```python
from build123d import *

# Parameters (mm, degrees)
SKETCH1_W           = 101.6
SKETCH1_H           = 101.6
BOSS_EXTRUDE2_DEPTH = 116.84
SKETCH2_W           = 76.2
SKETCH2_H           = 55.88
CUT_EXTRUDE1_DEPTH  = 99.06
SKETCH3_W           = 111.76
SKETCH3_H           = 17.78
CUT_EXTRUDE2_DEPTH  = 96.52
SKETCH4_W           = 96.52
SKETCH4_H           = 96.52
CUT_EXTRUDE3_DEPTH  = 35.56
SKETCH5_R           = 1.0795
BOSS_EXTRUDE3_DEPTH = 29.464
SKETCH8_W           = 3.048
SKETCH8_H           = 91.44
CUT_EXTRUDE4_DEPTH  = 2.54
SKETCH10_W          = 2.54
SKETCH10_H          = 5.08
SKETCH10_H_2        = 5.198880867
BOSS_EXTRUDE4_DEPTH = 96.52


with BuildPart() as part:
    # Sketch1 → Boss-Extrude2 (new body)
    with BuildSketch(Plane.XY):
        with Locations((50.8, -50.8)):
            Rectangle(SKETCH1_W, SKETCH1_H)
    extrude(amount=BOSS_EXTRUDE2_DEPTH)

    # Sketch2 → Cut-Extrude1 (cut)
    with BuildSketch(Plane(origin=(101.6, 0, 0), x_dir=(0, 0, -1), z_dir=(1, 0, 0))):
        with Locations((-40.64, -50.8)):
            Rectangle(SKETCH2_W, SKETCH2_H)
    extrude(amount=-CUT_EXTRUDE1_DEPTH, mode=Mode.SUBTRACT)

    # Sketch3 → Cut-Extrude2 (cut)
    with BuildSketch(Plane(origin=(99.06, 0, 0), x_dir=(0, 0, -1), z_dir=(1, 0, 0))):
        with Locations((-58.42, -90.17)):
            Rectangle(SKETCH3_W, SKETCH3_H)
        with Locations((-58.42, -11.43)):
            Rectangle(SKETCH3_W, SKETCH3_H)
    extrude(amount=-CUT_EXTRUDE2_DEPTH, mode=Mode.SUBTRACT)

    # Sketch4 → Cut-Extrude3 (cut)
    with BuildSketch(Plane.XY.offset(116.84)):
        with Locations((50.8, -50.8)):
            Rectangle(SKETCH4_W, SKETCH4_H)
    extrude(amount=-CUT_EXTRUDE3_DEPTH, mode=Mode.SUBTRACT)

    # Sketch5 → Boss-Extrude3 (add)
    with BuildSketch(Plane.XY.offset(81.28)):
        with Locations((85.09, -41.91)):
            Circle(SKETCH5_R)
        with Locations((85.09, -69.85)):
            Circle(SKETCH5_R)
        with Locations((34.29, -26.67)):
            Circle(SKETCH5_R)
        with Locations((33.02, -74.93)):
            Circle(SKETCH5_R)
    extrude(amount=BOSS_EXTRUDE3_DEPTH)

    # Sketch8 → Cut-Extrude4 (cut)
    with BuildSketch(Plane.ZY):
        with Locations((112.776, -50.8)):
            Rectangle(SKETCH8_W, SKETCH8_H)
    extrude(amount=-CUT_EXTRUDE4_DEPTH, mode=Mode.SUBTRACT)

    # Sketch10 → Boss-Extrude4 (add)
    with BuildSketch(Plane(origin=(2.54, 0, 0), x_dir=(0, 0, -1), z_dir=(1, 0, 0))):
        with Locations((-115.57, -96.52)):
            Rectangle(SKETCH10_W, SKETCH10_H)
        with Locations((-109.982, -96.52)):
            Rectangle(SKETCH10_W, SKETCH10_H)
        with Locations((-115.57, -5.139440434)):
            Rectangle(SKETCH10_W, SKETCH10_H_2)
        with Locations((-109.982, -5.08)):
            Rectangle(SKETCH10_W, SKETCH10_H)
    extrude(amount=BOSS_EXTRUDE4_DEPTH)


solid = part.part
```
Work out the finished part from the listing and answer in its coordinate system (mm). A direction names the side the tool comes from. Coordinates: 2 decimals unless noted, no trailing zeros. Loops run counter-clockwise (first coordinate to the right, second up) from the corner with the lowest first, then second, coordinate; pieces in that order, holes last. Notation, with made-up numbers: M 46,-27 L 78,-27 A10 cw 78,-18 Z; hole C 51.25,59 d9. An arc over 180 degrees is marked long. Use CSV: the item, a comma, the result in double quotes. Start each with the question number.
(1) Given pin 1 Ø12 at (x, y) = (74, -37) entering from +Z; pin 2 Ø5.5 at (x, y) = (51, -15.5) entering from +Z; pin 3 Ø6 at (y, z) = (-48.5, 31) entering from +X, each flat-ended and moving along its own axis, determine where each tip first touches the part or whether it passes through.
(2) Find section C-C, the plane x = 91. Give the vertices of the cut face in (y, z).
(3) For a pull along Y with two mould halves and no side action, classify faces 4 (the face through (53, -78.74, 41)), 5 (the face through (50, 0, 58)), 6 (the face through (47, -96, 116.84)) as +Y half, -Y half, draft (parallel to the pull), parting line (faces both ways), or undercut.
(4) Find section B-B, the plane y = -35.5. Give the vertices of the cut face in (x, z).
(5) Find section D-D, the plane z = 40.5. Give the vertices of the cut face in (x, y).
(6) For faces 1 (the face through (53, -51, 2.54)), 2 (the face through (50, -50, 81.28)), 3 (the face through (50, -2.54, 56)), determine the directions among +Z, -Z, +X, -X, +Y, -Y from which every point of the face is accessible in a straight line to the end or side of a thin tool.
(7) Consider line 1 (Y direction, x = 10, z = 42.5); line 2 (Z direction, x = 33, y = -5.5); line 3 (X direction, y = -54, z = 91.5). Determine where each line is inside the solid, lowest interval first.
(8) Find section A-A, the plane z = 87. Give the vertices of the cut face in (x, y).
Recorded:
1,pin 1,"stops at z = 81.28"
1,pin 2,"stops at z = 2.54"
1,pin 3,"stops at x = 2.54"
2,outline,"M -101.6,0 L 0,0 L 0,116.84 L -7.74,116.84 L -7.74,114.3 L -2.54,114.3 L -2.54,111.25 L -7.62,111.25 L -7.62,108.71 L -2.54,108.71 L -2.54,2.54 L -20.32,2.54 L -20.32,81.28 L -81.28,81.28 L -81.28,2.54 L -99.06,2.54 L -99.06,108.71 L -93.98,108.71 L -93.98,111.25 L -99.06,111.25 L -99.06,114.3 L -93.98,114.3 L -93.98,116.84 L -101.6,116.84 Z; hole M -78.74,2.54 L -22.86,2.54 L -22.86,78.74 L -78.74,78.74 Z"
3,face 4,"undercut"
3,face 5,"+Y half"
3,face 6,"draft"
4,outline,"M 0,0 L 101.6,0 L 101.6,2.54 L 2.54,2.54 L 2.54,78.74 L 101.6,78.74 L 101.6,116.84 L 99.06,116.84 L 99.06,81.28 L 2.54,81.28 L 2.54,111.25 L 0,111.25 Z; M 0,114.3 L 2.54,114.3 L 2.54,116.84 L 0,116.84 Z"
5,outline,"M 0,-101.6 L 101.6,-101.6 L 101.6,-78.74 L 2.54,-78.74 L 2.54,-22.86 L 101.6,-22.86 L 101.6,0 L 0,0 Z; hole M 2.54,-99.06 L 99.06,-99.06 L 99.06,-81.28 L 2.54,-81.28 Z; hole M 2.54,-20.32 L 99.06,-20.32 L 99.06,-2.54 L 2.54,-2.54 Z"
6,face 1,"+X"
6,face 2,"+Z"
6,face 3,"none"
7,line 1,"y = -101.6 to -99.06, -81.28 to -78.74, -22.86 to -20.32, -2.54 to 0"
7,line 2,"z = 0 to 2.54, 108.71 to 111.25, 114.3 to 116.84"
7,line 3,"x = 0 to 2.54, 99.06 to 101.6"
8,outline,"M 0,-101.6 L 101.6,-101.6 L 101.6,0 L 0,0 Z; C 33.02,-74.93 d2.16; C 34.29,-26.67 d2.16; C 85.09,-69.85 d2.16; C 85.09,-41.91 d2.16; hole M 2.54,-99.06 L 99.06,-99.06 L 99.06,-2.54 L 2.54,-2.54 Z"
